Autodesk Inventor part; units mm, degrees
ref_plane "YZ Plane" through (0, 0, 0) normal (1, 0, 0) x (0, 1, 0)
ref_plane "XZ Plane" through (0, 0, 0) normal (0, 1, 0) x (-1, 0, 0)
ref_plane "XY Plane" through (0, 0, 0) normal (0, 0, 1) x (1, 0, 0)
sketch "Skizze1" plane through (0, 0, 0) normal (0, 0, 1) x (1, 0, 0)
  circle A0 centre (0, 0) radius 8
  line L0 (-5.5, 0) -> (5.5, 0) construction
  circle A1 centre (0, 0) radius 3
  circle A2 centre (0, 0) radius 1.5
  arc A3 (-1.118, 1) -> (1.118, 1) centre (0, 0) ccw construction
  line L1 (-1.118, 1) -> (1.118, 1)
  dimension "d3" = 3
  dimension "d0" = 16
  dimension "d1" = 11
  dimension "d2" = 6
  dimension "d4" = 2.5
extrude "Extrusion1" add sketch "Skizze1" along normal blind 2 contours A1 | A2 L1 | L1 A2
sketch "Skizze2" plane through (0, 0, 2) normal (0, 0, 1) x (1, 0, 0)
  circle A0 centre (0, 0) radius 1.5
extrude "Extrusion2" add sketch "Skizze2" along normal blind 1
sketch "Skizze3" plane through (0, 0, 3) normal (0, 0, 1) x (1, 0, 0)
  circle A0 centre (0, 0) radius 1.5
  line L0 (-1.118, 1) -> (1.118, 1)
  circle A1 centre (0, 0) radius 1.5
extrude "Extrusion3" add sketch "Skizze3" along normal blind 7 contours A0 L0 picked at (0.0594, 0.1702)
extrude "Extrusion4" add sketch "Skizze1" against normal blind 16.75 contours A0 | A1 | A2 L1 | L1 A2
sketch "Skizze4" plane through (0, 0, -16.75) normal (0, 0, -1) x (-1, 0, 0)
  circle A0 centre (0, 0) radius 8
  arc A1 (-4.5, 6) -> (-4.5, -6) centre (0, 0) ccw
  arc A2 (4.5, -6) -> (4.5, 6) centre (0, 0) ccw
  line L0 (-4.5, 6) -> (4.5, 6)
  line L1 (4.5, -6) -> (-4.5, -6)
  dimension "d14" = 7.5
  dimension "d15" = 12
extrude "Extrusion5" add sketch "Skizze4" along normal blind 26.9 contours L0 A2 L1 A1
hole "Bohrung1" at (-5.5, 0, 0) at (5.5, 0, 0) direction (0, 0, -1) diameter 1.567 depth 3 tip angle 118
properties part number "DC-Motor_12V_150U-min" material "Aluminium 6061"
Could you check a few things on this model? Use its own coordinates, in mm. A direction names the side the tool comes from. Coordinates: 2 decimals unless noted, no trailing zeros. Write each loop counter-clockwise with the first axis right and the second up, starting at its lowest first coordinate (ties: lowest second). Pieces come first, ordered by that corner, then holes. Notation, with made-up numbers: (58.5, 39) -> (77.5, 39) arc R11 cw to (77.5, 46) -> close; hole circle Ø6 at (-31.5, -25.75). An arc over 180 degrees is marked (long way). Write item = value, one per line. Start each with the question number.
(1) I want a section at D-D (z = 1). Please give me the cut outline in (x, y), plus the area to 3 significant figures.
(2) I need wall thicknesses on line 1 (Z direction, x = -7, y = -1.25); line 2 (Y direction, x = 2, z = -23.5). Which ranges of each line are inside material? Lowest first, please. Write a range as [from, to].
(3) Which directions (+Z, -Z, +X, -X, +Y, -Y) give clear straight access to the entire face, cutting with the end or side of a thin tool? Please do faces 1 (the face through (0, 6, -30)), 2 (the face through (-7.5, 0.1, -30)), 3 (the face through (1.3, -1.3, 2)), 4 (the face through (0, -6.5, -16.75)).
(4) Will these pins go through, and if not, where does the flat tip stop? pin 1 (4.5 mm diameter, centred on x = -2, z = -36, fed in from +Y); pin 2 (8 mm diameter, centred on y = -6, z = -13.5, fed in from -X); pin 3 (1.8 mm diameter, centred on x = -0.5, z = 5, fed in from +Y).
(5) I want a section at A-A (x = 0). Please give me the cut outline in (y, z).
(6) I want a section at B-B (z = -9). Please give me the cut outline in (x, y).
(7) I want a section at C-C (y = 7). Please give me the cut outline in (x, z).
(8) We'd pull the mould along Y, two halves only. Please class faces 5 (the face through (0, 1, 6)), 6 (the face through (0, 0, 10)), 7 (the face through (4.723, 0.102, -1.521)): released by +Y, released by -Y, zero draft, split by the parting line, or undercut.
Result set:
q1.outline = circle Ø6 at (0, 0)
q1.area = 28.3 mm2
q2.line_1 = [-43.65, 0]
q2.line_2 = [-6, 6]
q3.face_1 = -Z, +X, -X, +Y
q3.face_2 = -Z, -X
q3.face_3 = +Z
q3.face_4 = -Z
q4.pin_1 = 6
q4.pin_2 = -7.75
q4.pin_3 = 1
q5.outline = (-8, -16.75) -> (-6, -16.75) -> (-6, -43.65) -> (6, -43.65) -> (6, -16.75) -> (8, -16.75) -> (8, 0) -> (3, 0) -> (3, 2) -> (1.5, 2) -> (1.5, 3) -> (1, 3) -> (1, 10) -> (-1.5, 10) -> (-1.5, 2) -> (-3, 2) -> (-3, 0) -> (-8, 0) -> close
q6.outline = circle Ø16 at (0, 0)
q7.outline = (-3.87, -16.75) -> (3.87, -16.75) -> (3.87, 0) -> (-3.87, 0) -> close
q8.face_5 = released by +Y
q8.face_6 = zero draft
q8.face_7 = undercut
